from build123d import *

# Parameters (mm, degrees)
F0_W      = 320
F0_H      = 420
F1_DEPTH  = 4
F3_DEPTH  = 4
F4_R      = 3
F5_DEPTH  = 25
F6_R      = 3
F7_DEPTH  = 25
F8_R      = 3
F9_DEPTH  = 25
F11_DEPTH = 25
F13_DEPTH = 25


with BuildPart() as f1:
    # F0 (on Top) → F1 (new body)
    with BuildSketch(Plane.XY):
        with Locations((160, 210)):
            Rectangle(F0_W, F0_H)
    extrude(amount=F1_DEPTH)

    # F2 (on face) → F3 (cut, through all)
    with BuildSketch(Plane.XY.offset(4)):
        Polygon((320, 420), (290, 420), (320, 360), align=None)
        Polygon((320, 60), (290, 0), (320, 0), align=None)
        with BuildLine():
            Line((113, 360), (213, 360))
            ThreePointArc((213, 360), (216.535534, 361.464466), (218, 365))
            Line((218, 365), (218, 403))
            ThreePointArc((218, 403), (216.535534, 406.535534), (213, 408))
            Line((213, 408), (113, 408))
            ThreePointArc((113, 408), (109.464466, 406.535534), (108, 403))
            Line((108, 403), (108, 365))
            ThreePointArc((108, 365), (109.464466, 361.464466), (113, 360))
        make_face()
        with BuildLine():
            Line((113, 12), (213, 12))
            ThreePointArc((213, 12), (216.535534, 13.464466), (218, 17))
            Line((218, 17), (218, 55))
            ThreePointArc((218, 55), (216.535534, 58.535534), (213, 60))
            Line((213, 60), (113, 60))
            ThreePointArc((113, 60), (109.464466, 58.535534), (108, 55))
            Line((108, 55), (108, 17))
            ThreePointArc((108, 17), (109.464466, 13.464466), (113, 12))
        make_face()
        Polygon((0, 420), (0, 210), (50, 420), align=None)
        Polygon((50, 0), (0, 210), (0, 0), align=None)
    extrude(amount=-F3_DEPTH, mode=Mode.SUBTRACT)

    # F4 (on face) → F5 (cut)
    with BuildSketch(Plane.XY.offset(4)):
        with Locations((67, 6)):
            Circle(F4_R)
        with Locations((97, 6)):
            Circle(F4_R)
        with Locations((127, 6)):
            Circle(F4_R)
        with Locations((157, 6)):
            Circle(F4_R)
        with Locations((187, 6)):
            Circle(F4_R)
        with Locations((217, 6)):
            Circle(F4_R)
        with Locations((247, 6)):
            Circle(F4_R)
        with Locations((277, 6)):
            Circle(F4_R)
        with Locations((64, 66)):
            Circle(F4_R)
        with Locations((94, 66)):
            Circle(F4_R)
        with Locations((124, 66)):
            Circle(F4_R)
        with Locations((220, 66)):
            Circle(F4_R)
        with Locations((250, 66)):
            Circle(F4_R)
        with Locations((280, 66)):
            Circle(F4_R)
        with Locations((310, 66)):
            Circle(F4_R)
        with Locations((67, 414)):
            Circle(F4_R)
        with Locations((64, 354)):
            Circle(F4_R)
        with Locations((97, 414)):
            Circle(F4_R)
        with Locations((310, 354)):
            Circle(F4_R)
        with Locations((277, 414)):
            Circle(F4_R)
        with Locations((94, 354)):
            Circle(F4_R)
        with Locations((220, 354)):
            Circle(F4_R)
        with Locations((280, 354)):
            Circle(F4_R)
        with Locations((124, 354)):
            Circle(F4_R)
        with Locations((127, 414)):
            Circle(F4_R)
        with Locations((250, 354)):
            Circle(F4_R)
        with Locations((157, 414)):
            Circle(F4_R)
        with Locations((187, 414)):
            Circle(F4_R)
        with Locations((217, 414)):
            Circle(F4_R)
        with Locations((247, 414)):
            Circle(F4_R)
    extrude(amount=-F5_DEPTH, mode=Mode.SUBTRACT)

    # F6 (on face) → F7 (cut)
    with BuildSketch(Plane.XY.offset(4)):
        with Locations((121, 90)):
            Circle(F6_R)
        with Locations((121, 130)):
            Circle(F6_R)
        with Locations((121, 170)):
            Circle(F6_R)
        with Locations((206, 90)):
            Circle(F6_R)
        with Locations((206, 130)):
            Circle(F6_R)
        with Locations((206, 170)):
            Circle(F6_R)
        with Locations((291, 80)):
            Circle(F6_R)
        with Locations((291, 120)):
            Circle(F6_R)
        with Locations((291, 160)):
            Circle(F6_R)
        with Locations((121, 330)):
            Circle(F6_R)
        with Locations((121, 290)):
            Circle(F6_R)
        with Locations((206, 330)):
            Circle(F6_R)
        with Locations((206, 250)):
            Circle(F6_R)
        with Locations((291, 340)):
            Circle(F6_R)
        with Locations((121, 250)):
            Circle(F6_R)
        with Locations((206, 290)):
            Circle(F6_R)
        with Locations((291, 300)):
            Circle(F6_R)
        with Locations((291, 260)):
            Circle(F6_R)
    extrude(amount=-F7_DEPTH, mode=Mode.SUBTRACT)

    # F8 (on face) → F9 (cut)
    with BuildSketch(Plane.XY.offset(4)):
        with Locations((15, 210)):
            Circle(F8_R)
        with Locations((45, 210)):
            Circle(F8_R)
    extrude(amount=-F9_DEPTH, mode=Mode.SUBTRACT)

    # F10 (on face) → F11 (intersect)
    with BuildSketch(Plane.XY.offset(4)):
        with BuildLine():
            Line((87, 350), (87, 355))
            ThreePointArc((87, 355), (85.535534, 358.535534), (82, 360))
            Line((82, 360), (57, 360))
            ThreePointArc((57, 360), (53.464466, 358.535534), (52, 355))
            Line((52, 355), (52, 340))
            ThreePointArc((52, 340), (50.535534, 336.464466), (47, 335))
            Line((47, 335), (0, 335))
            Line((0, 335), (0, 210))
            Line((0, 210), (0, 85))
            Line((0, 85), (47, 85))
            ThreePointArc((47, 85), (50.535534, 83.535534), (52, 80))
            Line((52, 80), (52, 65))
            ThreePointArc((52, 65), (53.464466, 61.464466), (57, 60))
            Line((57, 60), (82, 60))
            ThreePointArc((82, 60), (85.535534, 61.464466), (87, 65))
            Line((87, 65), (87, 70))
            ThreePointArc((87, 70), (88.464466, 73.535534), (92, 75))
            Line((92, 75), (275, 75))
            ThreePointArc((275, 75), (278.535534, 76.464466), (280, 80))
            Line((280, 80), (280, 82))
            ThreePointArc((280, 82), (281.464466, 85.535534), (285, 87))
            Line((285, 87), (320, 87))
            Line((320, 87), (320, 210))
            Line((320, 210), (320, 333))
            Line((320, 333), (285, 333))
            ThreePointArc((285, 333), (281.464466, 334.464466), (280, 338))
            Line((280, 338), (280, 340))
            ThreePointArc((280, 340), (278.535534, 343.535534), (275, 345))
            Line((275, 345), (92, 345))
            ThreePointArc((92, 345), (88.464466, 346.464466), (87, 350))
        make_face()
    extrude(amount=-F11_DEPTH, mode=Mode.INTERSECT)

    # F12 (on face) → F13 (cut)
    with BuildSketch(Plane.XY.offset(4)):
        with BuildLine():
            Line((320, 75), (320, 345))
            Line((320, 345), (200, 345))
            Line((200, 345), (200, 265))
            ThreePointArc((200, 265), (201.464466, 261.464466), (205, 260))
            Line((205, 260), (210, 260))
            ThreePointArc((210, 260), (213.535534, 258.535534), (215, 255))
            Line((215, 255), (215, 165))
            ThreePointArc((215, 165), (213.535534, 161.464466), (210, 160))
            Line((210, 160), (205, 160))
            ThreePointArc((205, 160), (201.464466, 158.535534), (200, 155))
            Line((200, 155), (200, 75))
            Line((200, 75), (320, 75))
        make_face()
    extrude(amount=-F13_DEPTH, mode=Mode.SUBTRACT)


solid = f1.part
CAD build for the part. Positions are in the model's coordinates, mm. Coordinates: 2 decimals unless noted, no trailing zeros. Write each loop counter-clockwise with the first axis right and the second up, starting at its lowest first coordinate (ties: lowest second). Pieces come first, ordered by that corner, then holes. Notation, with made-up numbers: M 43.5,61 L 47.5,61 A22 cw 47.5,68 Z; hole C 22.5,-9.75 d4. An arc over 180 degrees is marked long. Answer as a JSON object with one key per item and string values. Group by question number.
1) Saw through at C-C (y = 170). Write the cut outline in (x, z), plus the area to 3 significant figures.
2) Wall check: line 1 (Y direction, x = 206, z = 1.45); line 2 (X direction, y = 170, z = 2.55); line 3 (X direction, y = 354, z = 3.1). Give the ranges that are in metal, low to high. Write a range as from..to.
3) Saw through at B-B (y = 290). Write the cut outline in (x, z).
4) Saw through at D-D (z = 2.85). Give the number of separate pieces and of enclosed holes in the cut face, plus the area to 3 significant figures.
5) Mould opens along Y. For faces 1 (the face through (122.384, 87.338, 2.028)), 2 (the face through (15, 147, 2)), 3 (the face through (106, 212, 0)), 4 (the face through (206, 173, 2)) say: +Y half, -Y half, draft (parallel to the pull), parting line (faces both ways), or undercut.
6) Saw through at A-A (x = 64). Write the cut outline in (y, z).
7) Pin check, flat tips, straight feed: pin 1 Ø2 at (y, z) = (73.5, 2.5) entering from -X; pin 2 Ø1.5 at (y, z) = (316.5, 0.5) entering from -X; pin 3 Ø2 at (y, z) = (194.5, 1.5) entering from -X. Stop position of each tip, or through.
Values follow:
{
 "1": {"outline": "M 9.52,0 L 118,0 L 118,4 L 9.52,4 Z; M 124,0 L 203,0 L 203,4 L 124,4 Z; M 209,0 L 215,0 L 215,4 L 209,4 Z", "area": "774 mm2"},
 "2": {"line 1": "y = 160..167, 173..247, 253..260", "line 2": "x = 9.52..118, 124..203, 209..215", "line 3": "x = 52..61, 67..87"},
 "3": {"outline": "M 19.05,0 L 118,0 L 118,4 L 19.05,4 Z; M 124,0 L 200,0 L 200,4 L 124,4 Z"},
 "4": {"separate pieces": "1", "enclosed holes": "12", "area": "51,500 mm2"},
 "5": {"face 1": "undercut", "face 2": "-Y half", "face 3": "draft", "face 4": "undercut"},
 "6": {"outline": "M 60,0 L 63,0 L 63,4 L 60,4 Z; M 69,0 L 351,0 L 351,4 L 69,4 Z; M 357,0 L 360,0 L 360,4 L 357,4 Z"},
 "7": {"pin 1": "stops at x = 52", "pin 2": "stops at x = 25.18", "pin 3": "stops at x = 3.45"}
}
